Work out the finished part from the listing and answer in its coordinate system (mm). A direction names the side the tool comes from. Round coordinates to 2 decimals unless told otherwise and drop trailing zeros. Loops run counter-clockwise (first coordinate to the right, second up) from the corner with the lowest first, then second, coordinate; pieces in that order, holes last.
```python
from build123d import *

# Parameters (mm, degrees)
PAD_DEPTH      = 5
SKETCH001_W    = 15
SKETCH001_H    = 5
PAD001_DEPTH   = 10
SKETCH002_W    = 15
SKETCH002_H    = 5
PAD002_DEPTH   = 10
SKETCH003_W    = 15
SKETCH003_H    = 5
PAD003_DEPTH   = 10
SKETCH004_W    = 15
SKETCH004_H    = 55
PAD004_DEPTH   = 10
SKETCH005_R    = 1.7
HOLE_DEPTH     = 25
HOLE_TIPS_R    = 1.7
SKETCH006_W    = 15
SKETCH006_H    = 55
PAD005_DEPTH   = 10
SKETCH007_R    = 1.7
HOLE001_DEPTH  = 25
HOLE001_TIPS_R = 1.7
SKETCH008_W    = 15
SKETCH008_H    = 55
PAD006_DEPTH   = 10
SKETCH009_R    = 1.7
HOLE002_DEPTH  = 25
HOLE002_TIPS_R = 1.7


with BuildPart() as part:
    # Sketch → Pad (new body)
    with BuildSketch(Plane.XY):
        Polygon((77.465972, -44.725), (77.465972, -9.995), (87.465972, -9.995), (87.465972, -50.494492), (0, -100.995), (-87.465972, -50.494492), (-87.465972, 50.494492), (0, 100.995), (100.998008, 100.995), (188.464849, 50.495996), (180.578715, 36.836812), (89.45, 89.45), (0, 89.45), (-77.465972, 44.725), (-77.465972, -44.725), (0, -89.45), align=None)
    extrude(amount=PAD_DEPTH)

    # Sketch001 (on Face12 of Pad) → Pad001 (join)
    with BuildSketch(Plane.YZ.offset(87.465972)):
        with Locations((-30.244746, 2.5)):
            Rectangle(SKETCH001_W, SKETCH001_H)
    extrude(amount=PAD001_DEPTH)

    # Sketch002 (on Face19 of Pad001) → Pad002 (join)
    with BuildSketch(Plane(origin=(43.732986, -75.744746, 0), x_dir=(0.866017, 0.500015, 0), z_dir=(0.500015, -0.866017, 0))):
        with Locations((0, 2.5)):
            Rectangle(SKETCH002_W, SKETCH002_H)
    extrude(amount=PAD002_DEPTH)

    # Sketch003 (on Face22 of Pad002) → Pad003 (join)
    with BuildSketch(Plane(origin=(-43.732986, -75.744746, 0), x_dir=(0.866017, -0.500015, 0), z_dir=(-0.500015, -0.866017, 0))):
        with Locations((0, 2.5)):
            Rectangle(SKETCH003_W, SKETCH003_H)
    extrude(amount=PAD003_DEPTH)

    # Sketch004 (on Face30 of Pad003) → Pad004 (join)
    with BuildSketch(Plane.YZ.offset(97.465972)):
        with Locations((-30.244746, -22.5)):
            Rectangle(SKETCH004_W, SKETCH004_H)
    extrude(amount=PAD004_DEPTH)

    # Sketch005 (on Face41 of Pad004) → Hole (cut)
    with BuildSketch(Plane.YZ.offset(107.465972)):
        with Locations((-30.244746, -37.5)):
            Circle(SKETCH005_R)
        with Locations((-30.244746, -12.5)):
            Circle(SKETCH005_R)
    extrude(amount=-HOLE_DEPTH, mode=Mode.SUBTRACT)

    # Hole tips → Hole tip 1 section 0
    with BuildSketch(Plane.YZ.offset(82.465972), mode=Mode.PRIVATE) as hole_tip_1_s0:
        with Locations((-30.244746, -37.5)):
            Circle(HOLE_TIPS_R)
    loft([hole_tip_1_s0.sketch, Vertex(81.444509, -30.244746, -37.5)], mode=Mode.SUBTRACT)

    # Hole tips → Hole tip 2 section 0
    with BuildSketch(Plane.YZ.offset(82.465972), mode=Mode.PRIVATE) as hole_tip_2_s0:
        with Locations((-30.244746, -12.5)):
            Circle(HOLE_TIPS_R)
    loft([hole_tip_2_s0.sketch, Vertex(81.444509, -30.244746, -12.5)], mode=Mode.SUBTRACT)

    # Sketch006 (on Face33 of Hole) → Pad005 (join)
    with BuildSketch(Plane(origin=(48.733135, -84.404914, 0), x_dir=(0.866017, 0.500015, 0), z_dir=(0.500015, -0.866017, 0))):
        with Locations((0, -22.5)):
            Rectangle(SKETCH006_W, SKETCH006_H)
    extrude(amount=PAD005_DEPTH)

    # Sketch007 (on Face48 of Pad005) → Hole001 (cut)
    with BuildSketch(Plane(origin=(53.733284, -93.065082, 0), x_dir=(0.866017, 0.500015, 0), z_dir=(0.500015, -0.866017, 0))):
        with Locations((0, -37.5)):
            Circle(SKETCH007_R)
        with Locations((0, -12.5)):
            Circle(SKETCH007_R)
    extrude(amount=-HOLE001_DEPTH, mode=Mode.SUBTRACT)

    # Hole001 tips → Hole001 tip 1 section 0
    with BuildSketch(Plane(origin=(41.232912, -71.414662, 0), x_dir=(0.866017, 0.500015, 0), z_dir=(0.500015, -0.866017, 0)), mode=Mode.PRIVATE) as hole001_tip_1_s0:
        with Locations((0, -37.5)):
            Circle(HOLE001_TIPS_R)
    loft([hole001_tip_1_s0.sketch, Vertex(40.722165, -70.530058, -37.5)], mode=Mode.SUBTRACT)

    # Hole001 tips → Hole001 tip 2 section 0
    with BuildSketch(Plane(origin=(41.232912, -71.414662, 0), x_dir=(0.866017, 0.500015, 0), z_dir=(0.500015, -0.866017, 0)), mode=Mode.PRIVATE) as hole001_tip_2_s0:
        with Locations((0, -12.5)):
            Circle(HOLE001_TIPS_R)
    loft([hole001_tip_2_s0.sketch, Vertex(40.722165, -70.530058, -12.5)], mode=Mode.SUBTRACT)

    # Sketch008 (on Face36 of Hole001) → Pad006 (join)
    with BuildSketch(Plane(origin=(-48.733135, -84.404914, 0), x_dir=(0.866017, -0.500015, 0), z_dir=(-0.500015, -0.866017, 0))):
        with Locations((0, -22.5)):
            Rectangle(SKETCH008_W, SKETCH008_H)
    extrude(amount=PAD006_DEPTH)

    # Sketch009 (on Face55 of Pad006) → Hole002 (cut)
    with BuildSketch(Plane(origin=(-53.733284, -93.065082, 0), x_dir=(0.866017, -0.500015, 0), z_dir=(-0.500015, -0.866017, 0))):
        with Locations((0, -12.5)):
            Circle(SKETCH009_R)
        with Locations((0, -37.5)):
            Circle(SKETCH009_R)
    extrude(amount=-HOLE002_DEPTH, mode=Mode.SUBTRACT)

    # Hole002 tips → Hole002 tip 1 section 0
    with BuildSketch(Plane(origin=(-41.232912, -71.414662, 0), x_dir=(0.866017, -0.500015, 0), z_dir=(-0.500015, -0.866017, 0)), mode=Mode.PRIVATE) as hole002_tip_1_s0:
        with Locations((0, -12.5)):
            Circle(HOLE002_TIPS_R)
    loft([hole002_tip_1_s0.sketch, Vertex(-40.722165, -70.530058, -12.5)], mode=Mode.SUBTRACT)

    # Hole002 tips → Hole002 tip 2 section 0
    with BuildSketch(Plane(origin=(-41.232912, -71.414662, 0), x_dir=(0.866017, -0.500015, 0), z_dir=(-0.500015, -0.866017, 0)), mode=Mode.PRIVATE) as hole002_tip_2_s0:
        with Locations((0, -37.5)):
            Circle(HOLE002_TIPS_R)
    loft([hole002_tip_2_s0.sketch, Vertex(-40.722165, -70.530058, -37.5)], mode=Mode.SUBTRACT)


solid = part.part
```
1. Given pin 1 (7.5 mm diameter, centred on y = -26.5, z = -34, fed in from +X); pin 2 (6 mm diameter, centred on x = 97.5, z = -20, fed in from -Y); pin 3 (1.5 mm diameter, centred on y = -44.5, z = 1.5, fed in from +X), each flat-ended and moving along its own axis, determine where each tip first touches the part or whether it passes through.
Answer key:
pin 1: stops at x = 107.47
pin 2: stops at y = -37.74
pin 3: stops at x = 87.47
2. Find section C-C (y = 58). Write down the section's boundary in (x, z).
Answer key:
outline: (-74.47, 0) - (-54.47, 0) - (-54.47, 5) - (-74.47, 5) - close; (143.92, 0) - (175.47, 0) - (175.47, 5) - (143.92, 5) - close
3. Find section D-D (y = 34). Write down the section's boundary in (x, z), then the cut area to 3 significant figures.
Answer key:
outline: (-87.47, 0) - (-77.47, 0) - (-77.47, 5) - (-87.47, 5) - close
area: 50.0 mm2
4. Consider probe 1 along X at (y, z) = (-23, -26.5); probe 2 along Z at (x, y) = (111.5, 77); probe 3 along Y at (x, z) = (100, -12). Determine where each line is inside the solid, lowest interval first.
Answer key:
probe 1: x = 97.47 to 107.47
probe 2: z = 0 to 5
probe 3: y = -37.74 to -31.87, -28.62 to -22.74
5. Find section A-A (z = -43.5). Write down the section's boundary in (x, y).
Answer key:
outline: (-60.23, -89.31) - (-47.24, -96.82) - (-42.24, -88.16) - (-55.23, -80.65) - close; (42.24, -88.16) - (47.24, -96.82) - (60.23, -89.31) - (55.23, -80.65) - close; (97.47, -37.74) - (107.47, -37.74) - (107.47, -22.74) - (97.47, -22.74) - close
6. Which of the six approach directions +Z, -Z, +X, -X, +Y, -Y give full straight-line access (tool end or side, diameter ignored) to faces 4 (the face through (-68.586, -61.395, 2.465)), 5 (the face through (18.88, -90.094, 2.465)), 6 (the face through (102, -22.745, -23)), 7 (the face through (-38.19, 67.4, 2.46)), 8 (the face through (102, -37.745, -23))?
Answer key:
face 4: +Z, -Z, -X
face 5: +Z, -Z, -Y
face 6: +Z, -Z, +X
face 7: +Z, -Z
face 8: +Z, -Z, +X, -Y
7. Determine the mould class of faces 1 (the face through (82, -14, 0)), 2 (the face through (-44.35, 75.39, 2.46)), 3 (the face through (-52.74, -87.95, -12.43)) for opening direction Z: +Z half, -Z half, draft (parallel to the pull), parting line (faces both ways), or undercut.
Answer key:
face 1: -Z half
face 2: draft
face 3: undercut
8. Find section B-B (x = -24). Write down the section's boundary in (y, z).
Answer key:
outline: (-87.14, 0) - (-75.59, 0) - (-75.59, 5) - (-87.14, 5) - close; (75.59, 0) - (87.14, 0) - (87.14, 5) - (75.59, 5) - close
